Autodesk Inventor part; units mm, degrees
ref_plane "YZ Plane" through (0, 0, 0) normal (1, 0, 0) x (0, 1, 0)
ref_plane "XZ Plane" through (0, 0, 0) normal (0, 1, 0) x (-1, 0, 0)
ref_plane "XY Plane" through (0, 0, 0) normal (0, 0, 1) x (1, 0, 0)
sketch "Sketch1" plane through (0, 0, 0) normal (0, 0, 1) x (1, 0, 0)
  circle A0 centre (0, 0) radius 15.24
  dimension "d0" = 30.48
extrude "Extrusion1" add sketch "Sketch1" along normal mid plane 34.925
sketch "Sketch2" plane through (0, 0, -17.4625) normal (0, 0, -1) x (-1, 0, 0)
  circle A0 centre (0, 0) radius 15.24 construction
  circle A1 centre (0, 0) radius 16.51
  dimension "d5" = 33.02
extrude "Extrusion2" add sketch "Sketch2" along normal blind 3.175
sketch "Sketch3" plane through (0, 0, 17.4625) normal (0, 0, 1) x (1, 0, 0)
  circle A0 centre (0, 0) radius 15.24 construction
  circle A1 centre (0, 0) radius 6.35
  line L0 (-1.5875, 7.7359) -> (1.5875, 7.7359)
  line L1 (1.5875, 7.7359) -> (1.5875, 4.5609)
  line L2 (1.5875, 4.5609) -> (-1.5875, 4.5609)
  line L3 (-1.5875, 4.5609) -> (-1.5875, 7.7359)
  point P0 (0, 7.7359)
  point P1 (-1.5875, 6.1484)
  dimension "d8" = 12.7
  dimension "d9" = 3.175
  dimension "d10" = 3.175
extrude "Extrusion3" cut sketch "Sketch3" against normal through all
chamfer "Chamfer1" distance 1.5875 angle 45 1 edges at (-15.24, 0, 17.4625)
properties part number "LM Colson Hub 500 key" material "Aluminum 6061"
The model under review builds one solid part; all positions refer to its coordinate system, in mm. A direction names the side the tool comes from. Round coordinates to 2 decimals unless told otherwise and drop trailing zeros. Loops run counter-clockwise (first coordinate to the right, second up) from the corner with the lowest first, then second, coordinate; pieces in that order, holes last. Notation, with made-up numbers: M 6,8.25 L 47,8.25 A34 ccw 47,38.25 Z; hole C 89,12.5 d4. An arc over 180 degrees is marked long. Answer as a JSON object with one key per item and string values.
(1) Clearance check with flat-ended pins moving along their axes: P1, Ø2, axis at x = -9.5, z = 12, coming from the -Y side; P2, Ø1.5, axis at y = 2, z = -10, coming from the +X side; P3, Ø10, axis at x = 4.5, z = 3.5, coming from the -Y side. State where each tip first meets the part, or that it passes through.
Resolved:
{"P1": "y = -12.65", "P2": "x = 15.19", "P3": "y = -15.24"}
(2) Tool access review of faces 5 (the flat face through (0, -7, -20.638)), 6 (the flat face through (1.588, 7, -1)), 7 (the flat face through (-5, -15, -17.462)): name each direction out of +Z, -Z, +X, -X, +Y, -Y from which nothing blocks a thin tool from reaching the whole face with its end or side.
Resolved:
{"face 5": "-Z, +X, -X, +Y, -Y", "face 6": "+Z, -Z", "face 7": "+Z"}
(3) Draft analysis for pull direction X (two halves, no side actions). For faces 1 (the flat face through (0, 7.736, -1)), 2 (the flat face through (-1.588, 7, -1)), 3 (the cylindrical face through (-3.3, -14.88, -0.56)), 4 (the flat face through (6, -3, 17.462)), state which applies: released by +X, released by -X, zero draft, split by the parting line, or undercut.
Resolved:
{"face 1": "undercut", "face 2": "undercut", "face 3": "split by the parting line", "face 4": "zero draft"}
(4) To check wall thickness, follow line 1 along Y through (x, z) = (0, -3); line 2 along Z through (x, y) = (-12, -9.5); line 3 along X through (y, z) = (6.5, -10.5). State the ranges of each line that lie inside material, in increasing order.
Resolved:
{"line 1": "-15.24 to -6.35, 7.74 to 15.24", "line 2": "-20.64 to -17.46", "line 3": "-13.78 to -1.59, 1.59 to 13.78"}
(5) Take a section at C-C on z = 6. Give the boundary of the cut face in (x, y), and give its area (3 significant figures).
Resolved:
{"outline": "C 0,0 d30.48; hole M -1.59,6.15 A6.35 ccw long 1.59,6.15 L 1.59,7.74 L -1.59,7.74 Z", "area": "598 mm²"}
